Read the model definition and answer for the solid it produces. Units are mm, in the model's axes. Give positions to 0.01 mm unless a question says otherwise; leave off trailing zeros. Loops run counter-clockwise (first coordinate to the right, second up) from the corner with the lowest first, then second, coordinate; pieces in that order, holes last. Notation, with made-up numbers: (31.25, 55) -> (77.25, 55) arc R22 ccw to (77.25, 74) -> close; hole circle Ø6 at (71, 88.5). An arc over 180 degrees is marked (long way). Answer as CSV lines item,"result". Start each with the question number.
```python
from build123d import *

# Parameters (mm, degrees)
SKETCH1_W           = 3.175
SKETCH1_H           = 25.4
BOSS_EXTRUDE1_DEPTH = 3.175


with BuildPart() as part:
    # Sketch1 → Boss-Extrude1 (new body)
    with BuildSketch(Plane.XY):
        Polygon((406.4, 0), (406.4, 131.2672), (393.7, 131.2672), (393.7, 134.4422), (381, 134.4422), (381, 131.2672), (367.392857143, 131.2672), (367.392857143, 134.4422), (354.692857143, 134.4422), (354.692857143, 131.2672), (341.085714286, 131.2672), (341.085714286, 134.4422), (328.385714286, 134.4422), (328.385714286, 131.2672), (314.778571429, 131.2672), (314.778571429, 134.4422), (302.078571429, 134.4422), (302.078571429, 131.2672), (288.471428571, 131.2672), (288.471428571, 134.4422), (275.771428571, 134.4422), (275.771428571, 131.2672), (262.164285714, 131.2672), (262.164285714, 134.4422), (249.464285714, 134.4422), (249.464285714, 131.2672), (235.857142857, 131.2672), (235.857142857, 134.4422), (223.157142857, 134.4422), (223.157142857, 131.2672), (209.55, 131.2672), (209.55, 134.4422), (196.85, 134.4422), (196.85, 131.2672), (183.242857143, 131.2672), (183.242857143, 134.4422), (170.542857143, 134.4422), (170.542857143, 131.2672), (156.935714286, 131.2672), (156.935714286, 134.4422), (144.235714286, 134.4422), (144.235714286, 131.2672), (130.628571429, 131.2672), (130.628571429, 134.4422), (117.928571429, 134.4422), (117.928571429, 131.2672), (104.321428571, 131.2672), (104.321428571, 134.4422), (91.621428571, 134.4422), (91.621428571, 131.2672), (78.014285714, 131.2672), (78.014285714, 134.4422), (65.314285714, 134.4422), (65.314285714, 131.2672), (51.707142857, 131.2672), (51.707142857, 134.4422), (39.007142857, 134.4422), (39.007142857, 131.2672), (25.4, 131.2672), (25.4, 134.4422), (12.7, 134.4422), (12.7, 131.2672), (0, 131.2672), (0, 0), (12.7, 0), (12.7, -3.175), (25.4, -3.175), (25.4, 0), (39.007142857, 0), (39.007142857, -3.175), (51.707142857, -3.175), (51.707142857, 0), (65.314285714, 0), (65.314285714, -3.175), (78.014285714, -3.175), (78.014285714, 0), (91.621428571, 0), (91.621428571, -3.175), (104.321428571, -3.175), (104.321428571, 0), (117.928571429, 0), (117.928571429, -3.175), (130.628571429, -3.175), (130.628571429, 0), (144.235714286, 0), (144.235714286, -3.175), (156.935714286, -3.175), (156.935714286, 0), (170.542857143, 0), (170.542857143, -3.175), (183.242857143, -3.175), (183.242857143, 0), (196.85, 0), (196.85, -3.175), (209.55, -3.175), (209.55, 0), (223.157142857, 0), (223.157142857, -3.175), (235.857142857, -3.175), (235.857142857, 0), (249.464285714, 0), (249.464285714, -3.175), (262.164285714, -3.175), (262.164285714, 0), (275.771428571, 0), (275.771428571, -3.175), (288.471428571, -3.175), (288.471428571, 0), (302.078571429, 0), (302.078571429, -3.175), (314.778571429, -3.175), (314.778571429, 0), (328.385714286, 0), (328.385714286, -3.175), (341.085714286, -3.175), (341.085714286, 0), (354.692857143, 0), (354.692857143, -3.175), (367.392857143, -3.175), (367.392857143, 0), (381, 0), (381, -3.175), (393.7, -3.175), (393.7, 0), align=None)
        with Locations((4.7625, 91.0336)):
            Rectangle(SKETCH1_W, SKETCH1_H, mode=Mode.SUBTRACT)
        with Locations((4.7625, 40.2336)):
            Rectangle(SKETCH1_W, SKETCH1_H, mode=Mode.SUBTRACT)
        with Locations((401.6375, 91.0336)):
            Rectangle(SKETCH1_W, SKETCH1_H, mode=Mode.SUBTRACT)
        with Locations((401.6375, 40.2336)):
            Rectangle(SKETCH1_W, SKETCH1_H, mode=Mode.SUBTRACT)
    extrude(amount=BOSS_EXTRUDE1_DEPTH)


solid = part.part
```
(1) Each of these flat-tipped pins is pushed along its axis until it touches: P1, Ø1.5, axis at x = 191.5, z = 0.5, coming from the -Y side; P2, Ø1.6, axis at y = -2, z = 2, coming from the +X side; P3, Ø1, axis at y = 132, z = 1.5, coming from the -X side. Where does it stop, or does it pass through?
(2) Find section C-C on x = 321. Write down the section's boundary in (y, z) (3 decimals).
(3) Find the intervals of material crossed by line 1 along X through (y, z) = (49.5, 0.6) (3 decimals); line 2 along Y through (x, z) = (26, 1), in increasing order. Write a range as from..to.
(4) Find section B-B on z = 1.6. Give the number of separate pieces and of enclosed holes in the cut face, then the cut area to 3 significant figures.
(5) Find section A-A on y = 95. Write down the section's boundary in (x, z) (3 decimals), then the cut area to 3 significant figures.
Answer block:
1,P1,"stops at y = 0"
1,P2,"stops at x = 393.7"
1,P3,"stops at x = 12.7"
2,outline,"(0, 0) -> (131.267, 0) -> (131.267, 3.175) -> (0, 3.175) -> close"
3,line 1,"x = 0..3.175, 6.35..400.05, 403.225..406.4"
3,line 2,"y = 0..131.27"
4,separate pieces,"1"
4,enclosed holes,"4"
4,area,"54,200 mm2"
5,outline,"(0, 0) -> (3.175, 0) -> (3.175, 3.175) -> (0, 3.175) -> close; (6.35, 0) -> (400.05, 0) -> (400.05, 3.175) -> (6.35, 3.175) -> close; (403.225, 0) -> (406.4, 0) -> (406.4, 3.175) -> (403.225, 3.175) -> close"
5,area,"1,270 mm2"
